```python
from build123d import *

# Parameters (mm, degrees)
SKETCH1_W           = 30
SKETCH1_H           = 31
BOSS_EXTRUDE1_DEPTH = 2
SKETCH2_R           = 1
CUT_EXTRUDE2_DEPTH  = 4
FILLET2_R           = 5
FILLET3_R           = 5


with BuildPart() as part:
    # Sketch1 → Boss-Extrude1 (new body)
    with BuildSketch(Plane(origin=(0, 0, 0), x_dir=(1, 0, 0), z_dir=(0, 1, 0))):
        with Locations((-2.326732673, -4.50990099)):
            Rectangle(SKETCH1_W, SKETCH1_H)
    extrude(amount=BOSS_EXTRUDE1_DEPTH)

    # Sketch2 → Cut-Extrude2 (cut)
    with BuildSketch(Plane(origin=(0, 0, 0), x_dir=(1, 0, 0), z_dir=(0, 1, 0))):
        with Locations(Location((-9.826732673, 3.49009901, 0), (0, 0, 270))):
            Circle(SKETCH2_R)
        with Locations(Location((-9.826732673, -11.50990099, 0), (0, 0, 270))):
            Circle(SKETCH2_R)
        with Locations(Location((5.173267327, 3.49009901, 0), (0, 0, 270))):
            Circle(SKETCH2_R)
        with Locations(Location((5.173267327, -11.50990099, 0), (0, 0, 270))):
            Circle(SKETCH2_R)
    extrude(amount=CUT_EXTRUDE2_DEPTH, mode=Mode.SUBTRACT)

    # Fillet2
    # the kernel refuses this fillet: 5 mm, written as the material it takes off along each edge
    with BuildSketch(Plane(origin=(22.673267327, 2, 20.00990099), x_dir=(0, 0, -1), z_dir=(-1, 0, 0))) as fillet2_piece_1:
        with BuildLine():
            CenterArc((4, 5), FILLET2_R, 216.869897646, 53.130102354)
            Line((0, 2), (-0.08, 1.94))
            ThreePointArc((-0.08, 1.94), (-0.1, 1), (-0.1, 0))
            Line((-0.1, 0), (0, -0.1))
            Line((0, -0.1), (4, -0.1))
            Line((4, -0.1), (4, 0))
        make_face()
    extrude(amount=50, mode=Mode.SUBTRACT)

    # Fillet3
    # the kernel refuses this fillet: 5 mm, written as the material it takes off along each edge
    with BuildSketch(Plane(origin=(-27.326732673, 2, -10.99009901), x_dir=(0, -1, 0), z_dir=(1, 0, 0))) as fillet3_piece_1:
        with BuildLine():
            CenterArc((5, -4), FILLET3_R, 126.869897646, 53.130102354)
            Line((0, -4), (-0.1, -4))
            Line((-0.1, -4), (-0.1, 0))
            Line((-0.1, 0), (0, 0.1))
            ThreePointArc((0, 0.1), (1, 0.1), (1.94, 0.08))
            Line((1.94, 0.08), (2, 0))
        make_face()
    extrude(amount=50, mode=Mode.SUBTRACT)


solid = part.part
```
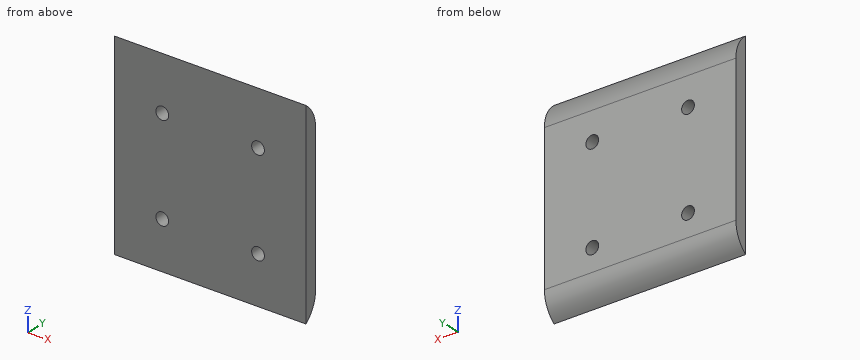
Work out the finished part from the listing and answer in its coordinate system (mm). Round coordinates to 2 decimals unless told otherwise and drop trailing zeros. Order: outer loops, then holes, each group sorted by start corner. A loop starts at its lowest first (then second) coordinate and runs counter-clockwise, first axis right, second up.
Q1. A cutting plane is placed at B-B, the plane y = 1.45. Determine the outline of the cut face in (x, z).
Solution:
outline: (-17.33, -9.27) - (12.67, -9.27) - (12.67, 18.29) - (-17.33, 18.29) - close; hole circle Ø2 at (-9.83, -3.49); hole circle Ø2 at (-9.83, 11.51); hole circle Ø2 at (5.17, -3.49); hole circle Ø2 at (5.17, 11.51)
Q2. A cutting plane is placed at C-C, the plane x = -2.25. Determine the outline of the cut face in (y, z), then the cut area to 3 significant figures.
Solution:
outline: (0, -10.99) arc R5 ccw to (2, -6.99) - (2, 16.01) arc R5 ccw to (0, 20.01) - close
area: 57.2 mm2
Q3. A cutting plane is placed at A-A, the plane x = 4.75. Determine the outline of the cut face in (y, z).
Solution:
outline: (0, -10.99) arc R5 ccw to (2, -6.99) - (2, -4.4) - (0, -4.4) - close; (0, -2.58) - (2, -2.58) - (2, 10.6) - (0, 10.6) - close; (0, 12.42) - (2, 12.42) - (2, 16.01) arc R5 ccw to (0, 20.01) - close
Q4. Given pin 1 Ø3 at (x, z) = (-4, 11.5) entering from -Y, flat-ended and moving along its own axis, determine where the tip first touches the part or whether it passes through.
Solution:
pin 1: stops at y = 0
Q5. Find the intervals of material crossed by line 1 along X through (y, z) = (1.2, -4); line 2 along Z through (x, y) = (4.5, 0.7); line 3 along Z through (x, y) = (-10, 1.25), in increasing order.
Solution:
line 1: x = -17.33 to -10.69, -8.97 to 4.31, 6.03 to 12.67
line 2: z = -10.35 to -4.23, -2.75 to 10.77, 12.25 to 19.37
line 3: z = -9.62 to -4.47, -2.51 to 10.53, 12.49 to 18.64
Q6. A cutting plane is placed at D-D, the plane z = -9. Determine the outline of the cut face in (x, y), then the cut area to 3 significant figures.
Solution:
outline: (-17.33, 0) - (12.67, 0) - (12.67, 1.58) - (-17.33, 1.58) - close
area: 47.3 mm2
